Can you work these out from the model? Positions are in its coordinate system, mm. A direction names the side the tool comes from. Coordinates: 2 decimals unless noted, no trailing zeros. Order: outer loops, then holes, each group sorted by start corner. A loop starts at its lowest first (then second) coordinate and runs counter-clockwise, first axis right, second up. Notation, with made-up numbers: (-18.5, 81) -> (10.5, 81) arc R25 cw to (10.5, 114) -> close; hole circle Ø5 at (-9.5, -9). An arc over 180 degrees is marked (long way). Write item = value, one per line. Start each with the question number.
from build123d import *

# Parameters (mm, degrees)
SKETCH028_W        = 89
SKETCH028_H        = 39
PAD015_DEPTH       = 64
SKETCH029_W        = 43
SKETCH029_H        = 39
POCKET011_DEPTH    = 3
CHAMFER_SIZE       = 2
SKETCH030_R        = 27.5
POCKET012_DEPTH    = 39.001
SKETCH031_W        = 15
SKETCH031_H        = 39
POCKET002_DEPTH    = 15
CHAMFER001_SIZE    = 14
SKETCH032_R        = 3.5
POCKET003_DEPTH    = 64.001
BODY007_ROLL_ANGLE = 90


with BuildPart() as part:
    # Sketch028 → Pad015 (new body)
    with BuildSketch(Plane.XY):
        Rectangle(SKETCH028_W, SKETCH028_H)
    extrude(amount=PAD015_DEPTH)

    # Sketch029 → Pocket011 (cut)
    with BuildSketch(Plane.XY):
        Rectangle(SKETCH029_W, SKETCH029_H)
    extrude(amount=POCKET011_DEPTH, mode=Mode.SUBTRACT)

    # Chamfer
    chamfer_edges = [part.edges().sort_by_distance(p)[0] for p in [
        (21.5, 0, 0),
        (-21.5, 0, 0),
        (44.5, 0, 0),
        (-44.5, 0, 0),
    ]]
    chamfer(chamfer_edges, length=CHAMFER_SIZE)

    # Sketch030 (on Face1 of Chamfer) → Pocket012 (cut, through all)
    with BuildSketch(Plane.XZ.offset(19.5)):
        with Locations((0, 34.5)):
            Circle(SKETCH030_R)
    extrude(amount=-POCKET012_DEPTH, mode=Mode.SUBTRACT)

    # Sketch031 (on Face7 of Pocket012) → Pocket002 (cut)
    with BuildSketch(Plane.XY.offset(64)):
        with Locations((-37, 0)):
            Rectangle(SKETCH031_W, SKETCH031_H)
        with Locations((37, 0)):
            Rectangle(SKETCH031_W, SKETCH031_H)
    extrude(amount=-POCKET002_DEPTH, mode=Mode.SUBTRACT)

    # Chamfer001
    chamfer001_edges = [part.edges().sort_by_distance(p)[0] for p in [
        (29.5, 0, 64),
        (-29.5, 0, 64),
    ]]
    chamfer(chamfer001_edges, length=CHAMFER001_SIZE)

    # Sketch032 (on Face10 of Chamfer001) → Pocket003 (cut, through all)
    with BuildSketch(Plane(origin=(0, 0, 0), x_dir=(1, 0, 0), z_dir=(0, 0, -1))):
        with Locations((-35, -10)):
            Circle(SKETCH032_R)
        with Locations((-35, 10)):
            Circle(SKETCH032_R)
        with Locations((35, 10)):
            Circle(SKETCH032_R)
        with Locations((35, -10)):
            Circle(SKETCH032_R)
    extrude(amount=-POCKET003_DEPTH, mode=Mode.SUBTRACT)


with BuildPart() as part_1:
    # Body007 roll: moved
    add(part.part.rotate(Axis((0, 0, 0), (1, 0, 0)), BODY007_ROLL_ANGLE))


with BuildPart() as part_2:
    # Body007 placement: moved
    add(part_1.part.moved(Location((0, -30, 32))))


solid = part_2.part
(1) For faces 1 (the face through (37, -79, 32)), 2 (the face through (32.42, -54.157, 19.635)), 3 (the face through (22.5, -31, 31.7)), 4 (the face through (-37, -79, 32)), which set-ups out of +Z, -Z, +X, -X, +Y, -Y let a thin tool reach every point of the face, with its end or its side?
(2) Imagine slicing it at B-B (y = -81). Write out the boundary of the cut face in (x, z), plus the area to 3 significant figures.
(3) Imagine slicing it at A-A (z = 42). Write out the boundary of the cut face in (x, y).
(4) Thinking about a two-plate mould opening in Z: for faces 5 (the face through (19, -40, 12.5)), 6 (the face through (-35.46, -54.16, 38.53)), 7 (the face through (-3.58, -91.766, 31.727)), which applies, +Z half, -Z half, draft (parallel to the pull), parting line (faces both ways), or undercut?
(5) Imagine slicing it at C-C (x = 0). Write out the boundary of the cut face in (y, z), plus the area to 3 significant figures.
(6) If I drill on L1, parallel to Z at x = -35, y = -48; L2, parallel to X at y = -41, z = 21; L3, parallel to Z at x = -34, y = -61.5, over which ranges is the centre line in solid material (lowest first)? Write a range as from..to.
(7) For P1, Ø5.5, axis at x = -35, z = 22, coming from the +Y side; P2, Ø9, axis at x = 35, z = 22, coming from the -Y side; P3, Ø4, axis at x = -28.5, z = 42.5, coming from the -Y side; P4, Ø0.8, axis at y = -79.5, z = 27, coming from the +X side, each with a flat end and sliding along its axis, tell me the tip position at first contact or that it passes through.
(8) Imagine slicing it at D-D (x = 35). Write out the boundary of the cut face in (y, z).
Result set:
q1.face_1 = +Z, -Z, +X, -Y
q1.face_2 = +Y, -Y
q1.face_3 = +Z, -Z, +Y
q1.face_4 = +Z, -Z, -X, -Y
q2.outline = (-28.5, 12.5) -> (-22, 12.5) -> (-22, 51.5) -> (-28.5, 51.5) -> close; (22, 12.5) -> (28.5, 12.5) -> (28.5, 51.5) -> (22, 51.5) -> close
q2.area = 507 mm2
q3.outline = (-44.5, -79) -> (-38.5, -79) -> (-38.5, -30) -> (-42.5, -30) -> (-44.5, -32) -> close; (-31.5, -79) -> (-29.5, -79) -> (-29.5, -80) -> (-15.5, -94) -> (15.5, -94) -> (29.5, -80) -> (29.5, -79) -> (31.5, -79) -> (31.5, -30) -> (23.5, -30) -> (21.5, -32) -> (21.5, -33) -> (-21.5, -33) -> (-21.5, -32) -> (-23.5, -30) -> (-31.5, -30) -> close; (38.5, -79) -> (44.5, -79) -> (44.5, -32) -> (42.5, -30) -> (38.5, -30) -> close; hole circle Ø55 at (0, -64.5)
q4.face_5 = -Z half
q4.face_6 = undercut
q4.face_7 = draft
q5.outline = (-94, 12.5) -> (-92, 12.5) -> (-92, 51.5) -> (-94, 51.5) -> close; (-37, 12.5) -> (-33, 12.5) -> (-33, 51.5) -> (-37, 51.5) -> close
q5.area = 234 mm2
q6.L1 = 12.5..18.5, 25.5..38.5, 45.5..51.5
q6.L2 = -44.5..-38.35, -31.65..-14.28, 14.28..31.65, 38.35..44.5
q6.L3 = 12.5..18.65, 25.35..38.65, 45.35..51.5
q7.P1 = through
q7.P2 = -79
q7.P3 = -83
q7.P4 = 29.5
q8.outline = (-79, 12.5) -> (-30, 12.5) -> (-30, 18.5) -> (-79, 18.5) -> close; (-79, 25.5) -> (-30, 25.5) -> (-30, 38.5) -> (-79, 38.5) -> close; (-79, 45.5) -> (-30, 45.5) -> (-30, 51.5) -> (-79, 51.5) -> close
